```python
from build123d import *

# Parameters (mm, degrees)
F1_DEPTH = 3.96875


with BuildPart() as f1:
    # F0 (on Top) → F1 (new body)
    with BuildSketch(Plane.XY):
        with BuildLine():
            ThreePointArc((6.327746, 3.651619), (5.817408, 5.040304), (4.842658, 6.153296))
            ThreePointArc((4.842658, 6.153296), (3.908213, 6.97687), (2.837203, 7.612792))
            ThreePointArc((2.837203, 7.612792), (1.455709, 8.435292), (0, 9.117891))
            ThreePointArc((0, 9.117891), (-2.984964, 7.632257), (-5.546768, 5.498181))
            ThreePointArc((-5.546768, 5.498181), (-6.145468, 4.663163), (-6.411583, 3.670753))
            ThreePointArc((-6.411583, 3.670753), (-5.947905, 0.406573), (-4.103787, -2.326392))
            ThreePointArc((-4.103787, -2.326392), (-2.598583, -5.259348), (-0.090588, -7.398935))
            ThreePointArc((-0.090588, -7.398935), (2.544544, -5.363511), (3.970517, -2.354611))
            ThreePointArc((3.970517, -2.354611), (5.704057, 0.406109), (6.357343, 3.599845))
            Line((6.357343, 3.599845), (6.327746, 3.651619))
        make_face()
    extrude(amount=F1_DEPTH)


solid = f1.part
```
Source: CAD feature listing. Evaluate the final solid. Frame: model axes, mm. Coordinates: 2 decimals unless noted, no trailing zeros. Loops run counter-clockwise (first coordinate to the right, second up) from the corner with the lowest first, then second, coordinate; pieces in that order, holes last. Notation, with made-up numbers: (71.5, 22) -> (110.5, 22) arc R25 cw to (110.5, 55) -> close; hole circle Ø1 at (-9.5, 13). An arc over 180 degrees is marked (long way). One line per item, written item: value. Start each with the question number.
Q1. Section query A-A, the plane z = 2.4. Return the cut outline in (x, y).
Q2. Section query C-C, the plane y = -5.25. Return the cut outline in (x, z), and give its area (3 significant figures).
Q3. Section query B-B, the plane x = 3.25. Return the cut outline in (y, z), and give its area (3 significant figures).
Q4. Line query: line 1 along X through (y, z) = (0.5, 2); line 2 along X through (y, z) = (0, 3.5); line 3 along Y through (x, z) = (2.5, 3.6). Output: solid intervals per line, ascending.
Q5. Contact query for a flat-ended pin moving along its axis: P1, Ø1.5, axis at y = 2.5, z = 3, coming from the +X side. Output: stop coordinate, or through.
Results:
1. outline: (-6.41, 3.67) arc R7.35 ccw to (-4.1, -2.33) arc R8.5 ccw to (-0.09, -7.4) arc R7.14 ccw to (3.97, -2.35) arc R9.13 ccw to (6.36, 3.6) -> (6.33, 3.65) arc R4.05 ccw to (4.84, 6.15) arc R6.68 ccw to (2.84, 7.61) arc R16.32 ccw to (0, 9.12) arc R14.36 ccw to (-5.55, 5.5) arc R2.87 ccw to start
2. outline: (-2.61, 0) -> (2.63, 0) -> (2.63, 3.97) -> (-2.61, 3.97) -> close
2. area: 20.8 mm^2
3. outline: (-4.31, 0) -> (7.4, 0) -> (7.4, 3.97) -> (-4.31, 3.97) -> close
3. area: 46.5 mm^2
4. line 1: -5.98 to 5.74
4. line 2: -5.78 to 5.53
4. line 3: -5.42 to 7.83
5. P1: x = 6.34
